Read the model definition and answer for the solid it produces. Units are mm, in the model's axes. Face numbers are marked on the shaded views. Round coordinates to 2 decimals unless told otherwise and drop trailing zeros. One line per item, written item: value. Start each with the question number.
1. Section A-A (y = 1.65) is taken. State how many separate pieces and enclosed holes the cut face has, then the cut area to 3 significant figures.
2. The mould has two halves that part along X. Classify the marked faces 1 and 2: released by +X, released by -X, zero draft, split by the parting line, or undercut.
3. A flat-ended cylindrical pin translates along its axis: pin 1 Ø1 at (x, z) = (0.5, 5.5) entering from +Y. Find the tip coordinate at first contact, or state that the pin passes through.
4. Consider line 1 (Y direction, x = 0, z = 5.25); line 2 (Z direction, x = -0.55, y = -1.05); line 3 (Y direction, x = 0.3, z = 0.5). Determine where each line is inside the solid, lowest interval first.
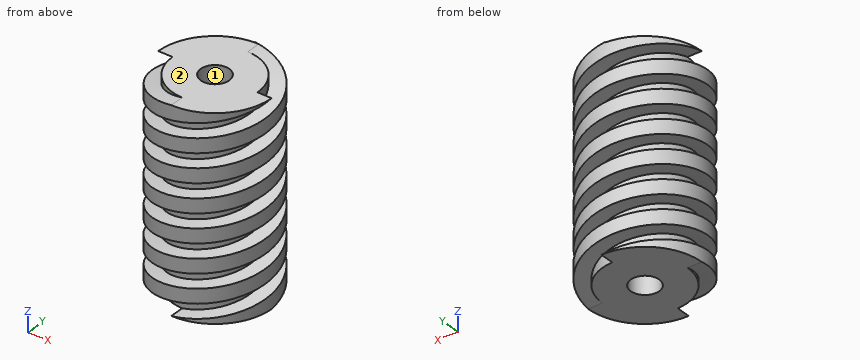
from build123d import *

# Parameters (mm, degrees)
SKETCH2_R               = 1.5
BOSS_EXTRUDE1_DEPTH     = 7
SWEEP1_PITCH            = 2
SWEEP1_HEIGHT           = 7.5
SWEEP1_RADIUS           = 2
SKETCH5_W               = 0.50487755
SKETCH5_H               = 0.5
SWEEP2_PITCH            = 2
SWEEP2_HEIGHT           = 7.5
SWEEP2_RADIUS           = 2
SWEEP2_START_ANGLE      = 180
SKETCH6_W               = 0.5
SKETCH6_H               = 0.5
CUT_EXTRUDE1_DEPTH      = 9.018050785
CUT_EXTRUDE1_DEPTH_BACK = 9.018050785
SKETCH8_W               = 0.5
SKETCH8_H               = 4
SKETCH8_H_2             = 4.221172624
SKETCH9_R               = 0.5
CUT_EXTRUDE2_DEPTH      = 8.552425988


with BuildPart() as part:
    # Sketch2 → Boss-Extrude1 (new body)
    with BuildSketch(Plane.XY):
        Circle(SKETCH2_R)
    extrude(amount=BOSS_EXTRUDE1_DEPTH)

    # Sweep1: sweep along a helix
    with BuildLine() as sweep1_path:
        Helix(SWEEP1_PITCH, SWEEP1_HEIGHT, SWEEP1_RADIUS, center=(0, 0, 7.5), direction=(0, 0, -1))
    # Sketch5 → Sweep1 (sweep)
    with BuildSketch(Plane(origin=(0, 0, 0), x_dir=(1, 0, 0), z_dir=(0, 1, 0))):
        with Locations((-1.752438775, -7.25)):
            Rectangle(SKETCH5_W, SKETCH5_H)
    sweep(path=sweep1_path.line, is_frenet=True)

    # Sweep2: sweep along a helix
    with BuildLine() as sweep2_path:
        add(Helix(SWEEP2_PITCH, SWEEP2_HEIGHT, SWEEP2_RADIUS, center=(0, 0, 7.5), direction=(0, 0, -1), mode=Mode.PRIVATE).rotate(Axis((0, 0, 7.5), (0, 0, -1)), SWEEP2_START_ANGLE))
    # Sketch6 → Sweep2 (sweep)
    with BuildSketch(Plane(origin=(0, 0, 0), x_dir=(1, 0, 0), z_dir=(0, 1, 0))):
        with Locations((1.75, -7.25)):
            Rectangle(SKETCH6_W, SKETCH6_H)
    sweep(path=sweep2_path.line, is_frenet=True)

    # Sketch8 → Cut-Extrude1 (cut, two sides: drawn at the far end of the back side and taken through both)
    with BuildSketch(Plane(origin=(0, 0, 0), x_dir=(0, 0, -1), z_dir=(1, 0, 0)).offset(-CUT_EXTRUDE1_DEPTH_BACK)):
        with Locations((-7.25, 0)):
            Rectangle(SKETCH8_W, SKETCH8_H)
        with Locations((0.25, -0.110586312)):
            Rectangle(SKETCH8_W, SKETCH8_H_2)
    extrude(amount=CUT_EXTRUDE1_DEPTH + CUT_EXTRUDE1_DEPTH_BACK, mode=Mode.SUBTRACT)

    # Sketch9 → Cut-Extrude2 (cut, through all)
    with BuildSketch(Plane.XY.offset(7)):
        Circle(SKETCH9_R)
    extrude(amount=-CUT_EXTRUDE2_DEPTH, mode=Mode.SUBTRACT)


solid = part.part
Answer:
1. separate pieces: 8
1. enclosed holes: 0
1. area: 7.94 mm^2
2. face 1: undercut
2. face 2: zero draft
3. pin 1: y = 2
4. line 1: -1.5 to -0.5, 0.5 to 1.5
4. line 2: 0 to 7
4. line 3: -1.47 to -0.4, 0.4 to 1.98
